Geometry check sheet. Reference: the model listing, model coordinates, mm. Give positions to 0.01 mm unless a question says otherwise; leave off trailing zeros. Loops run counter-clockwise (first coordinate to the right, second up) from the corner with the lowest first, then second, coordinate; pieces in that order, holes last. Notation, with made-up numbers: (-5, 40.25) - (50, 40.25) arc R17 cw to (50, 66.25) - close; hole circle Ø10 at (9.5, 25.25). An arc over 180 degrees is marked (long way). One line per question, with ' | ' between items. Start each with the question number.
Autodesk Inventor part; units mm, degrees
ref_plane "YZ Plane" through (0, 0, 0) normal (1, 0, 0) x (0, 1, 0)
ref_plane "XZ Plane" through (0, 0, 0) normal (0, 1, 0) x (-1, 0, 0)
ref_plane "XY Plane" through (0, 0, 0) normal (0, 0, 1) x (1, 0, 0)
sketch "Sketch1" plane through (0, 0, 0) normal (0, 0, 1) x (1, 0, 0)
  line L0 (-28.575, -9.525) -> (28.575, -9.525)
  line L1 (28.575, -9.525) -> (28.575, 9.525)
  line L2 (28.575, 9.525) -> (-28.575, 9.525)
  line L3 (-28.575, 9.525) -> (-28.575, -9.525)
  line L4 (-28.575, -9.525) -> (28.575, 9.525) construction
  line L5 (28.575, -9.525) -> (-28.575, 9.525) construction
  point P0 (0, 0)
  dimension "d0" = 57.15
  dimension "d1" = 19.05
extrude "Extrusion1" add sketch "Sketch1" against normal blind 4.7625
sketch "Sketch2" plane through (0, 0, 0) normal (0, 0, 1) x (1, 0, 0)
  line L0 (-28.575, -9.525) -> (-28.575, 9.525) construction
  line L1 (-28.575, 0) -> (28.575, 0) construction
  line L2 (28.575, 9.525) -> (28.575, -9.525) construction
  spline S0 degree 2 poles (-15.2755, 3.6741) (-14.7352, 3.0412) (-14.1331, 1.1887) (-14.1331, 0) knots 0 0 0 1 2 2 2
  spline S1 degree 2 poles (-14.1331, 0) (-14.1331, -1.1578) (-14.7198, -3.0335) (-15.2755, -3.6664) knots 0 0 0 1 2 2 2
  spline S2 degree 2 poles (-15.2755, -3.6664) (-15.8621, -4.3302) (-17.4136, -4.9632) (-18.3476, -4.9632) knots 0 0 0 1 2 2 2
  spline S3 degree 2 poles (-18.3476, -4.9632) (-19.3124, -4.9632) (-20.8562, -4.3071) (-21.4197, -3.6664) knots 0 0 0 1 2 2 2
  spline S4 degree 2 poles (-21.4197, -3.6664) (-21.9677, -3.0335) (-22.5543, -1.1733) (-22.5543, 0) knots 0 0 0 1 2 2 2
  spline S5 degree 2 poles (-22.5543, 0) (-22.5543, 1.1964) (-21.96, 3.0181) (-21.412, 3.6741) knots 0 0 0 1 2 2 2
  spline S6 degree 2 poles (-21.412, 3.6741) (-20.8562, 4.3071) (-19.3047, 4.9632) (-18.3476, 4.9632) knots 0 0 0 1 2 2 2
  spline S7 degree 2 poles (-18.3476, 4.9632) (-17.375, 4.9632) (-15.8158, 4.2839) (-15.2755, 3.6741) knots 0 0 0 1 2 2 2
  spline S8 degree 2 poles (-15.453, 0) (-15.453, 0.9417) (-15.8621, 2.4005) (-16.2326, 2.8791) knots 0 0 0 1 2 2 2
  spline S9 degree 2 poles (-16.2326, 2.8791) (-16.6109, 3.3731) (-17.6761, 3.8671) (-18.3399, 3.8671) knots 0 0 0 1 2 2 2
  spline S10 degree 2 poles (-18.3399, 3.8671) (-19.0268, 3.8671) (-20.0612, 3.3886) (-20.4548, 2.8791) knots 0 0 0 1 2 2 2
  spline S11 degree 2 poles (-20.4548, 2.8791) (-20.833, 2.3928) (-21.2344, 0.9263) (-21.2344, 0) knots 0 0 0 1 2 2 2
  spline S12 degree 2 poles (-21.2344, 0) (-21.2344, -1.8757) (-19.6598, -3.8671) (-18.3399, -3.8671) knots 0 0 0 1 2 2 2
  spline S13 degree 2 poles (-18.3399, -3.8671) (-17.02, -3.8671) (-15.453, -1.8757) (-15.453, 0) knots 0 0 0 1 2 2 2
  line L3 (-5.928, -4.7625) -> (-7.3483, -4.7625)
  line L4 (-7.3483, -4.7625) -> (-11.5628, 3.4503)
  line L5 (-11.5628, 3.4503) -> (-11.5628, -4.7625)
  line L6 (-11.5628, -4.7625) -> (-12.7437, -4.7625)
  line L7 (-12.7437, -4.7625) -> (-12.7437, 4.7625)
  line L8 (-12.7437, 4.7625) -> (-10.9453, 4.7625)
  line L9 (-10.9453, 4.7625) -> (-7.109, -2.7788)
  line L10 (-7.109, -2.7788) -> (-7.109, 4.7625)
  line L11 (-7.109, 4.7625) -> (-5.928, 4.7625)
  line L12 (-5.928, 4.7625) -> (-5.928, -4.7625)
  line L13 (-0.3088, 5.187) -> (-4.0369, -6.8311)
  line L14 (-4.0369, -6.8311) -> (-5.1176, -6.8311)
  line L15 (-5.1176, -6.8311) -> (-1.4048, 5.187)
  line L16 (-1.4048, 5.187) -> (-0.3088, 5.187)
  spline S14 degree 2 poles (7.7497, 3.6741) (8.29, 3.0412) (8.8921, 1.1887) (8.8921, 0) knots 0 0 0 1 2 2 2
  spline S15 degree 2 poles (8.8921, 0) (8.8921, -1.1578) (8.3054, -3.0335) (7.7497, -3.6664) knots 0 0 0 1 2 2 2
  spline S16 degree 2 poles (7.7497, -3.6664) (7.163, -4.3302) (5.6116, -4.9632) (4.6776, -4.9632) knots 0 0 0 1 2 2 2
  spline S17 degree 2 poles (4.6776, -4.9632) (3.7127, -4.9632) (2.169, -4.3071) (1.6055, -3.6664) knots 0 0 0 1 2 2 2
  spline S18 degree 2 poles (1.6055, -3.6664) (1.0575, -3.0335) (0.4708, -1.1733) (0.4708, 0) knots 0 0 0 1 2 2 2
  spline S19 degree 2 poles (0.4708, 0) (0.4708, 1.1964) (1.0652, 3.0181) (1.6132, 3.6741) knots 0 0 0 1 2 2 2
  spline S20 degree 2 poles (1.6132, 3.6741) (2.169, 4.3071) (3.7205, 4.9632) (4.6776, 4.9632) knots 0 0 0 1 2 2 2
  spline S21 degree 2 poles (4.6776, 4.9632) (5.6502, 4.9632) (7.2094, 4.2839) (7.7497, 3.6741) knots 0 0 0 1 2 2 2
  spline S22 degree 2 poles (7.5721, 0) (7.5721, 0.9417) (7.163, 2.4005) (6.7925, 2.8791) knots 0 0 0 1 2 2 2
  spline S23 degree 2 poles (6.7925, 2.8791) (6.4143, 3.3731) (5.3491, 3.8671) (4.6853, 3.8671) knots 0 0 0 1 2 2 2
  spline S24 degree 2 poles (4.6853, 3.8671) (3.9983, 3.8671) (2.964, 3.3886) (2.5704, 2.8791) knots 0 0 0 1 2 2 2
  spline S25 degree 2 poles (2.5704, 2.8791) (2.1921, 2.3928) (1.7908, 0.9263) (1.7908, 0) knots 0 0 0 1 2 2 2
  spline S26 degree 2 poles (1.7908, 0) (1.7908, -1.8757) (3.3654, -3.8671) (4.6853, -3.8671) knots 0 0 0 1 2 2 2
  spline S27 degree 2 poles (4.6853, -3.8671) (6.0052, -3.8671) (7.5721, -1.8757) (7.5721, 0) knots 0 0 0 1 2 2 2
  line L17 (15.9779, 3.6356) -> (11.5473, 3.6356)
  line L18 (11.5473, 3.6356) -> (11.5473, 0.9494)
  line L19 (11.5473, 0.9494) -> (15.7927, 0.9494)
  line L20 (15.7927, 0.9494) -> (15.7927, -0.1775)
  line L21 (15.7927, -0.1775) -> (11.5473, -0.1775)
  line L22 (11.5473, -0.1775) -> (11.5473, -4.7625)
  line L23 (11.5473, -4.7625) -> (10.2814, -4.7625)
  line L24 (10.2814, -4.7625) -> (10.2814, 4.7625)
  line L25 (10.2814, 4.7625) -> (15.9779, 4.7625)
  line L26 (15.9779, 4.7625) -> (15.9779, 3.6356)
  line L27 (22.8091, 3.6356) -> (18.3785, 3.6356)
  line L28 (18.3785, 3.6356) -> (18.3785, 0.9494)
  line L29 (18.3785, 0.9494) -> (22.6238, 0.9494)
  line L30 (22.6238, 0.9494) -> (22.6238, -0.1775)
  line L31 (22.6238, -0.1775) -> (18.3785, -0.1775)
  line L32 (18.3785, -0.1775) -> (18.3785, -4.7625)
  line L33 (18.3785, -4.7625) -> (17.1126, -4.7625)
  line L34 (17.1126, -4.7625) -> (17.1126, 4.7625)
  line L35 (17.1126, 4.7625) -> (22.8091, 4.7625)
  line L36 (22.8091, 4.7625) -> (22.8091, 3.6356)
  point P0 (0, 0)
extrude "Extrusion2" cut sketch "Sketch2" against normal blind 3.175
fillet "Fillet1" radius 1.5875 4 edges at (0, 9.525, 0) (28.575, 0, 0) (0, -9.525, 0) (-28.575, 0, 0)
equation "\"d0\" = width"
equation "\"d1\" = height"
equation "\"d2\" = depth"
equation "\"d13\" = textDepth"
equation "\"width\" = 57.15"
equation "\"height\" = 19.05"
equation "\"depth\" = 4.7625"
equation "\"textDepth\" = 0.666667 * depth"
properties part number "onOffSign"
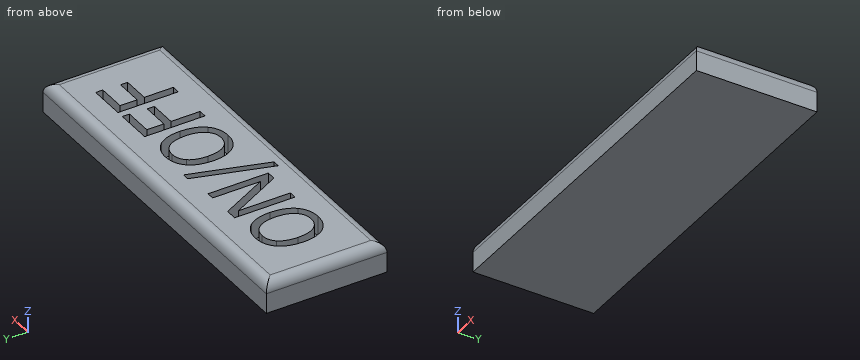
(1) Section check C-C, the plane x = -9.5. Record the boundary of the cut face in (y, z) (1 decimal), and give its area (3 significant figures).
(2) Section check B-B, the plane x = 11. Record the boundary of the cut face in (y, z) (1 decimal), and give its area (3 significant figures).
(3) Material ranges on line 1 (Y direction, x = 11, z = -2.55) (1 decimal); line 2 (X direction, y = -5.25, z = -1.1); line 3 (Z direction, x = -12, y = 3.5) (1 decimal), recorded low to high.
(4) Section check A-A, the plane x = 22. Record the boundary of the cut face in (y, z) (1 decimal).
(5) Depth check by flat-ended pin: pin 1 Ø4 at (x, y) = (17, -4) entering from +Z; pin 2 Ø0.9 at (x, z) = (-4.5, -1) entering from +Y. Enter the tip coordinate at first touch or a pass-through.
Numbers:
1) outline: (-9.5, -4.8) - (9.5, -4.8) - (9.5, -1.6) arc R1.6 ccw to (7.9, 0) - (1.9, 0) - (1.9, -3.2) - (-0.6, -3.2) - (-0.6, 0) - (-7.9, 0) arc R1.6 ccw to (-9.5, -1.6) - close | area: 81.7 mm^2
2) outline: (-9.5, -4.8) - (9.5, -4.8) - (9.5, -1.6) arc R1.6 ccw to (7.9, 0) - (4.8, 0) - (4.8, -3.2) - (-4.8, -3.2) - (-4.8, 0) - (-7.9, 0) arc R1.6 ccw to (-9.5, -1.6) - close | area: 59.4 mm^2
3) line 1: -9.5 to -4.8, 4.8 to 9.5 | line 2: -28.5 to -4.63, -3.55 to 28.5 | line 3: -4.8 to -3.2
4) outline: (-9.5, -4.8) - (9.5, -4.8) - (9.5, -1.6) arc R1.6 ccw to (7.9, 0) - (4.8, 0) - (4.8, -3.2) - (3.6, -3.2) - (3.6, 0) - (0.9, 0) - (0.9, -3.2) - (-0.2, -3.2) - (-0.2, 0) - (-7.9, 0) arc R1.6 ccw to (-9.5, -1.6) - close
5) pin 1: z = 0 | pin 2: y = 9.52
